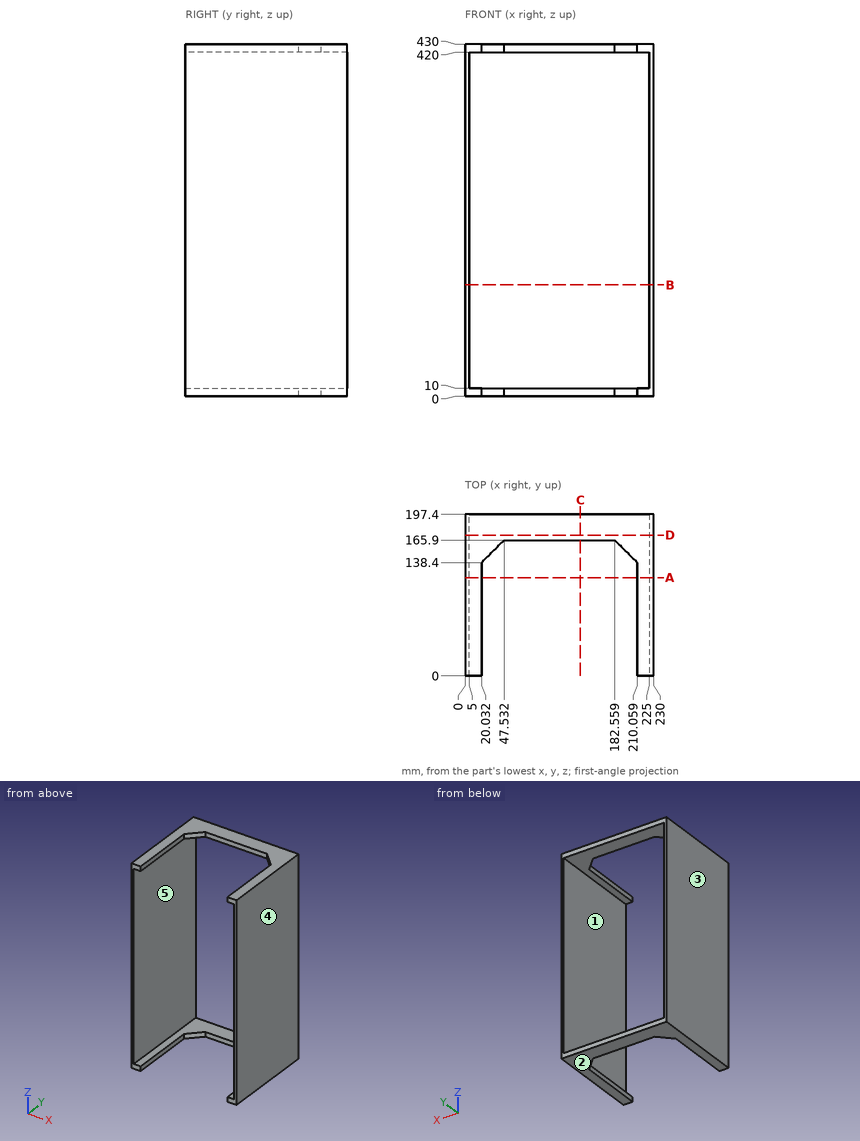
Part print with two shaded views. Sizes in mm from the minimum x, y, z corner. A direction names the side the tool comes from. Coordinates: 2 decimals unless noted, no trailing zeros. Write each loop counter-clockwise with the first axis right and the second up, starting at its lowest first coordinate (ties: lowest second). Pieces come first, ordered by that corner, then holes. Notation, with made-up numbers: (26, -38) -> (62, -38) arc R36 cw to (62, 0) -> close; hole circle Ø1 at (-4, 77.5). An arc over 180 degrees is marked (long way). Return JSON: item names as keys, results as strings. Group by question number.
Q1. Cut at C-C, the plane x = 140.5. Give the cut face in (y, z), then the cut area to 3 significant figures.
Q2. Pull direction Z, two halves, no side cores. Call the marked faces 1, 2 and 3: released by +Z, released by -Z, zero draft, split by the parting line, or undercut.
Q3. Which spindle directions (+Z, -Z, +X, -X, +Y, -Y) get a long thin tool onto all of the face, cutting with end or side? Do the marked faces 4 and 5. Say none if no direction does.
Q4. Flat gauge pin, fed straight in: pin 1 (8 mm diameter, centred on x = 100, z = 5.5, fed in from -Y). Where does the tip first touch, or does it go through?
Q5. Cut at D-D, the plane y = 172. Give the cut face in (x, z), then the cut area to 3 significant figures.
Q6. Cut at B-B, the plane z = 136. Give the cut face in (x, y).
Q7. Drill centre lines: line 1 (X direction, y = 67, z = 160); line 2 (Z direction, x = 215, y = 160). Where is each one in solid material? Low to high.
Q8. Cut at A-A, the plane y = 120. Give the cut face in (x, z), then the cut area to 3 significant figures.
Returned:
{
 "1": {"outline": "(165.9, 0) -> (197.4, 0) -> (197.4, 10) -> (165.9, 10) -> close; (165.9, 420) -> (197.4, 420) -> (197.4, 430) -> (165.9, 430) -> close", "area": "630 mm2"},
 "2": {"face 1": "undercut", "face 2": "released by -Z", "face 3": "zero draft"},
 "3": {"face 4": "+Z, -Z, +X, +Y, -Y", "face 5": "+Y, -Y"},
 "4": {"pin 1": "stops at y = 165.9"},
 "5": {"outline": "(0, 0) -> (230, 0) -> (230, 430) -> (0, 430) -> close; hole (5, 10) -> (225, 10) -> (225, 420) -> (5, 420) -> close", "area": "8,700 mm2"},
 "6": {"outline": "(0, 0) -> (5, 0) -> (5, 197.4) -> (0, 197.4) -> close; (225, 0) -> (230, 0) -> (230, 197.4) -> (225, 197.4) -> close"},
 "7": {"line 1": "x = 0 to 5, 225 to 230", "line 2": "z = 0 to 10, 420 to 430"},
 "8": {"outline": "(0, 0) -> (20.03, 0) -> (20.03, 10) -> (5, 10) -> (5, 420) -> (20.03, 420) -> (20.03, 430) -> (0, 430) -> close; (210.06, 0) -> (230, 0) -> (230, 430) -> (210.06, 430) -> (210.06, 420) -> (225, 420) -> (225, 10) -> (210.06, 10) -> close", "area": "4,900 mm2"}
}
